For this review, take the finished solid that the model builds, in its own axes (mm). Face numbers are marked on the shaded views. A direction names the side the tool comes from. Coordinates: 2 decimals unless noted, no trailing zeros. Order: outer loops, then holes, each group sorted by start corner. A loop starts at its lowest first (then second) coordinate and runs counter-clockwise, first axis right, second up.
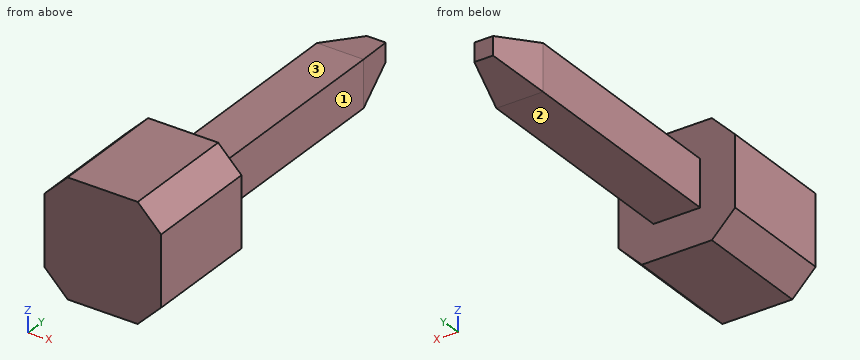
Autodesk Inventor part; units mm, degrees
ref_plane "YZ Plane" through (0, 0, 0) normal (1, 0, 0) x (0, 1, 0)
ref_plane "XZ Plane" through (0, 0, 0) normal (0, 1, 0) x (-1, 0, 0)
ref_plane "XY Plane" through (0, 0, 0) normal (0, 0, 1) x (1, 0, 0)
sketch "Sketch1" plane through (0, 0, 0) normal (0, 1, 0) x (-1, 0, 0)
  line L0 (-1.25, -1.25) -> (1.25, -1.25)
  line L1 (1.25, -1.25) -> (1.25, 1.25)
  line L2 (1.25, 1.25) -> (-1.25, 1.25)
  line L3 (-1.25, 1.25) -> (-1.25, -1.25)
  line L4 (-1.25, -1.25) -> (1.25, 1.25) construction
  line L5 (1.25, -1.25) -> (-1.25, 1.25) construction
  point P0 (0, 0)
  dimension "d0" = 2.5
  dimension "d1" = 2.5
extrude "Extrusion1" add sketch "Sketch1" along normal blind 2.5
chamfer "Chamfer1" distance 0.5 angle 45 4 edges at (1.25, 1.25, 1.25) (-1.25, 1.25, 1.25) (1.25, 1.25, -1.25) (-1.25, 1.25, -1.25)
sketch "Sketch2" plane through (0, 2.5, 0) normal (0, 1, 0) x (1, 0, 0)
  line L0 (-0.5, 0.5) -> (0.5, 0.5)
  line L1 (0.5, 0.5) -> (0.5, -0.5)
  line L2 (0.5, -0.5) -> (-0.5, -0.5)
  line L3 (-0.5, -0.5) -> (-0.5, 0.5)
  point P0 (0, 0)
  dimension "d7" = 1
  dimension "d9" = 1
  dimension "d10" = 0.5
  dimension "d11" = 0.5
extrude "Extrusion2" add sketch "Sketch2" along normal blind 6
chamfer "Chamfer2" distance 0.3 angle 75 4 edges at (0, 8.5, 0.5) (-0.5, 8.5, 0) (0, 8.5, -0.5) (0.5, 8.5, 0) measured on face at (-0.1667, 8.5, -0.1667)
properties part number "nanopc_t4_pin"
1. Machinability: for the marked faces 1, 2 and 3, which of the approach directions +Z, -Z, +X, -X, +Y, -Y give a long, thin tool a straight path to every point of the face, cutting with its end or side? Answer none if there is none.
Answer below:
face 1: +Z, -Z, +X, +Y
face 2: -Z, +X, -X, +Y
face 3: +Z, +X, -X, +Y
2. Take a section at C-C, the plane y = 3. Give the boundary of the cut face in (x, z), plus the area to 3 significant figures.
Answer below:
outline: (-0.5, -0.5) - (0.5, -0.5) - (0.5, 0.5) - (-0.5, 0.5) - close
area: 1.00 mm2
3. Take a section at A-A, the plane z = -0.4. Give the boundary of the cut face in (x, y), plus the area to 3 significant figures.
Answer below:
outline: (-1.25, 0) - (1.25, 0) - (1.25, 2.5) - (0.5, 2.5) - (0.5, 7.38) - (0.4, 7.75) - (-0.4, 7.75) - (-0.5, 7.38) - (-0.5, 2.5) - (-1.25, 2.5) - close
area: 11.5 mm2
4. Clearance check with flat-ended pins moving along their axes: pin 1 Ø1.5 at (y, z) = (6.5, -0.5) entering from +X; pin 2 Ø1 at (x, z) = (-0.5, 1) entering from -Y; pin 3 Ø0.5 at (x, y) = (0, 4.5) entering from -Z; pin 4 Ø0.5 at (x, y) = (0, 5.5) entering from +Z. State where each tip first meets the part, or that it passes through.
Answer below:
pin 1: stops at x = 0.5
pin 2: stops at y = 0
pin 3: stops at z = -0.5
pin 4: stops at z = 0.5
5. To check wall thickness, follow L1, parallel to Y at x = -1, z = -0.6; L2, parallel to X at y = 5.5, z = -0.3. State the ranges of each line that lie inside material, in increasing order.
Answer below:
L1: y = 0 to 2.5
L2: x = -0.5 to 0.5
6. Take a section at B-B, the plane x = -0.65. Give the boundary of the cut face in (y, z).
Answer below:
outline: (0, -1.25) - (2.5, -1.25) - (2.5, 1.25) - (0, 1.25) - close
7. Take a section at D-D, the plane z = 0.3. Give the boundary of the cut face in (x, y), plus the area to 3 significant figures.
Answer below:
outline: (-1.25, 0) - (1.25, 0) - (1.25, 2.5) - (0.5, 2.5) - (0.5, 7.38) - (0.3, 8.13) - (-0.3, 8.13) - (-0.5, 7.38) - (-0.5, 2.5) - (-1.25, 2.5) - close
area: 11.7 mm2
